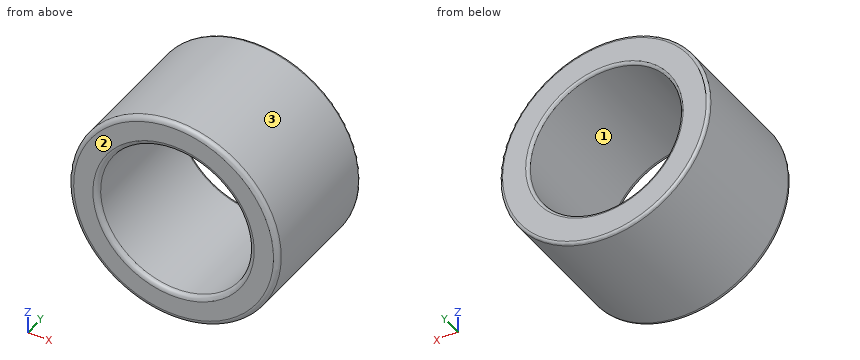
```python
from build123d import *

# Parameters (mm, degrees)
SKETCH1_R           = 10.87817
SKETCH1_R_2         = 7.87817
BOSS_EXTRUDE1_DEPTH = 14
FILLET1_R           = 0.3
FILLET5_R           = 0.3
FILLET6_R           = 0.5
FILLET7_R           = 0.5


with BuildPart() as part:
    # Sketch1 → Boss-Extrude1 (new body)
    with BuildSketch(Plane(origin=(0, 0, 0), x_dir=(1, 0, 0), z_dir=(0, 1, 0))):
        with Locations(Location((0, 0, 0), (0, 0, 270))):
            Circle(SKETCH1_R)
        with Locations(Location((0, 0, 0), (0, 0, 270))):
            Circle(SKETCH1_R_2, mode=Mode.SUBTRACT)
    extrude(amount=BOSS_EXTRUDE1_DEPTH)

    # Fillet1
    fillet1_edges = [part.edges().sort_by_distance(p)[0] for p in [
        (0, 14, -10.87817),
    ]]
    fillet(fillet1_edges, radius=FILLET1_R)

    # Fillet5
    fillet5_edges = [part.edges().sort_by_distance(p)[0] for p in [
        (0, 14, -7.87817),
    ]]
    fillet(fillet5_edges, radius=FILLET5_R)

    # Fillet6
    fillet6_edges = [part.edges().sort_by_distance(p)[0] for p in [
        (0, 0, -10.87817),
    ]]
    fillet(fillet6_edges, radius=FILLET6_R)

    # Fillet7
    fillet7_edges = [part.edges().sort_by_distance(p)[0] for p in [
        (0, 0, -7.87817),
    ]]
    fillet(fillet7_edges, radius=FILLET7_R)


solid = part.part
```
Input: part model. Units: mm. Frame: model coordinates. Face numbers are marked on the shaded views. Round coordinates to 2 decimals unless told otherwise and drop trailing zeros. Order: outer loops, then holes, each group sorted by start corner. A loop starts at its lowest first (then second) coordinate and runs counter-clockwise, first axis right, second up. Notation, with made-up numbers: (27, 57) - (33, 57) arc R30 ccw to (33, 81) - close; hole circle Ø7 at (56.25, 45). An arc over 180 degrees is marked (long way). Answer in a Markdown table with one row per item.
Item 1: Pin query (flat end, axial travel): pin 1 (3 mm diameter, centred on y = 2.5, z = -4, fed in from -X); pin 2 (5 mm diameter, centred on y = 2, z = 5.5, fed in from +X); pin 3 (4 mm diameter, centred on x = -7, y = 10, fed in from +Z). Return the tip coordinate at first contact, or that it passes through.
Model answer:
| item | result |
|---|---|
| pin 1 | stops at x = -10.59 |
| pin 2 | stops at x = 10.46 |
| pin 3 | stops at z = 9.66 |
Item 2: Mould query, pull axis X, two halves, no side actions, for the marked faces 1, 2 and 3. Classes: released by +X, released by -X, zero draft, split by the parting line, or undercut.
Model answer:
| item | result |
|---|---|
| face 1 | undercut |
| face 2 | zero draft |
| face 3 | split by the parting line |
Item 3: Section query B-B (z = 0). Return the cut outline in (x, y).
Model answer:
| item | result |
|---|---|
| outline | (-10.88, 0.5) arc R0.5 ccw to (-10.38, 0) - (-8.38, 0) arc R0.5 ccw to (-7.88, 0.5) - (-7.88, 13.7) arc R0.3 ccw to (-8.18, 14) - (-10.58, 14) arc R0.3 ccw to (-10.88, 13.7) - close; (7.88, 0.5) arc R0.5 ccw to (8.38, 0) - (10.38, 0) arc R0.5 ccw to (10.88, 0.5) - (10.88, 13.7) arc R0.3 ccw to (10.58, 14) - (8.18, 14) arc R0.3 ccw to (7.88, 13.7) - close |
Item 4: Section query A-A (x = 0). Return the cut outline in (y, z), then the cut area to 3 significant figures.
Model answer:
| item | result |
|---|---|
| outline | (0, -10.38) arc R0.5 ccw to (0.5, -10.88) - (13.7, -10.88) arc R0.3 ccw to (14, -10.58) - (14, -8.18) arc R0.3 ccw to (13.7, -7.88) - (0.5, -7.88) arc R0.5 ccw to (0, -8.38) - close; (0, 8.38) arc R0.5 ccw to (0.5, 7.88) - (13.7, 7.88) arc R0.3 ccw to (14, 8.18) - (14, 10.58) arc R0.3 ccw to (13.7, 10.88) - (0.5, 10.88) arc R0.5 ccw to (0, 10.38) - close |
| area | 83.7 mm² |
Item 5: Line query: line 1 (X direction, y = 3.75, z = 0); line 2 (Z direction, x = -0.25, y = 3.25); line 3 (Z direction, x = -6.5, y = 7.25). Output: solid intervals per line, ascending.
Model answer:
| item | result |
|---|---|
| line 1 | x = -10.88 to -7.88, 7.88 to 10.88 |
| line 2 | z = -10.88 to -7.87, 7.87 to 10.88 |
| line 3 | z = -8.72 to -4.45, 4.45 to 8.72 |
Item 6: Section query C-C (y = 9.5). Return the cut outline in (x, z).
Model answer:
| item | result |
|---|---|
| outline | circle Ø21.76 at (0, 0); hole circle Ø15.76 at (0, 0) |
